```python
from build123d import *
from build123d.topology import SkipClean

# Parameters (mm, degrees)
SKETCH1_R           = 30
BOSS_EXTRUDE1_DEPTH = 20
SKETCH2_R           = 27
CUT_EXTRUDE1_DEPTH  = 7
CUT_EXTRUDE2_START  = -9
SKETCH3_R           = 27
CUT_EXTRUDE2_DEPTH  = 9
SKETCH4_R           = 6
SKETCH4_R_2         = 4
BOSS_EXTRUDE2_DEPTH = 18
BOSS_EXTRUDE3_START = 2
SKETCH5_R           = 6
BOSS_EXTRUDE3_DEPTH = 2
CUT_EXTRUDE7_START  = -42
SKETCH6_R           = 4
CUT_EXTRUDE7_DEPTH  = 42
SKETCH7_W           = 3
SKETCH7_H           = 2
BOSS_EXTRUDE4_DEPTH = 20
CIRPATTERN1_COUNT   = 25


with BuildPart() as part:
    # Sketch1 → Boss-Extrude1 (new body)
    with BuildSketch(Plane.XY):
        Circle(SKETCH1_R)
    extrude(amount=BOSS_EXTRUDE1_DEPTH)

    # Sketch2 → Cut-Extrude1 (cut)
    with BuildSketch(Plane.XY.offset(20)):
        Circle(SKETCH2_R)
    extrude(amount=-CUT_EXTRUDE1_DEPTH, mode=Mode.SUBTRACT)

    # Sketch3 → Cut-Extrude2 (cut)
    with BuildSketch(Plane(origin=(0, 0, 0), x_dir=(-1, 0, 0), z_dir=(0, 0, -1)).offset(CUT_EXTRUDE2_START)):
        with Locations(Location((0, 0, 0), (0, 0, 180))):
            Circle(SKETCH3_R)
    extrude(amount=CUT_EXTRUDE2_DEPTH, mode=Mode.SUBTRACT)

    # Sketch4 → Boss-Extrude2 (add)
    with BuildSketch(Plane.XY.offset(13)):
        Circle(SKETCH4_R)
        Circle(SKETCH4_R_2, mode=Mode.SUBTRACT)
    extrude(amount=BOSS_EXTRUDE2_DEPTH)

    # Sketch5 → Boss-Extrude3 (add)
    with BuildSketch(Plane(origin=(0, 0, 9), x_dir=(-1, 0, 0), z_dir=(0, 0, -1)).offset(BOSS_EXTRUDE3_START)):
        with Locations(Location((0, 0, 0), (0, 0, 180))):
            Circle(SKETCH5_R)
    extrude(amount=-BOSS_EXTRUDE3_DEPTH)

    # Sketch6 → Cut-Extrude7 (cut)
    with SkipClean():  # the faces are left unmerged after this step: merging them gives an invalid solid
        with BuildSketch(Plane.XY.offset(31).offset(CUT_EXTRUDE7_START)):
            with Locations(Location((0, 0, 0), (0, 0, 180))):
                Circle(SKETCH6_R)
        extrude(amount=CUT_EXTRUDE7_DEPTH, mode=Mode.SUBTRACT)
    add(part.part.scale(1), mode=Mode.REPLACE)  # the faces are merged on a copy

    # Sketch7 → Boss-Extrude4 (add)
    with BuildSketch(Plane.XY.offset(20)):
        with Locations((0, 30.891402014)):
            Rectangle(SKETCH7_W, SKETCH7_H)
    boss_extrude4 = extrude(amount=-BOSS_EXTRUDE4_DEPTH)

    # CirPattern1: Boss-Extrude4 ×25 about axis
    cirpattern1_axis = Axis((0, 0, 0), (0, 0, 1))
    for i in range(1, CIRPATTERN1_COUNT):
        add(boss_extrude4.rotate(cirpattern1_axis, i * 360 / CIRPATTERN1_COUNT))


solid = part.part
```
The model under review builds one solid part; all positions refer to its coordinate system, in mm. A direction names the side the tool comes from. Coordinates: 2 decimals unless noted, no trailing zeros. Write each loop counter-clockwise with the first axis right and the second up, starting at its lowest first coordinate (ties: lowest second). Pieces come first, ordered by that corner, then holes. Notation, with made-up numbers: (50, 7.5) - (65, 7.5) arc R14 ccw to (65, 34.5) - close; hole circle Ø8 at (74, -32.75). An arc over 180 degrees is marked (long way). Write item = value, one per line.
(1) For line 1 (Y direction, x = 0, z = 16.75); line 2 (Y direction, x = -16.5, z = 14); line 3 (Z direction, x = -16, y = 21.5), list the stretches that pass through material, from the lowest coordinate up. Write a range as [from, to].
Result sheet:
line_1 = [-30, -27], [-6, -4], [4, 6], [27, 31.89]
line_2 = [-25.26, -21.37], [21.37, 25.05], [26.9, 27.32]
line_3 = [9, 13]
(2) For P1, Ø8, axis at x = 24, y = 1.5, coming from the -Z side; P2, Ø1, axis at x = 4.5, z = 17, coming from the +Y side; P3, Ø6, axis at x = 2, y = 1.5, coming from the -Z side; P4, Ø6, axis at y = -15.5, z = 11, coming from the -X side, all flat-tipped, find the tip position at first contact; note any pin that passes through.
Result sheet:
P1 = 0
P2 = 29.73
P3 = 7
P4 = -29.36
(3) Consider section B-B, the plane z = 15. State how many separate pieces and enclosed holes the cut face has, then the cut area to 3 significant figures.
Result sheet:
separate_pieces = 2
enclosed_holes = 2
area = 743 mm^2
(4) Machinability: for faces 1 (the face through (-0.4, 6.4, 13)), 2 (the face through (-23.095, 19.147, 9.86)), 3 (the face through (-12.775, -28.19, 10.14)), 4 (the face through (30.65, -4.32, 10.14)), which of the approach directions +Z, -Z, +X, -X, +Y, -Y give a long, thin tool a straight path to every point of the face, cutting with its end or side? Answer none if there is none.
Result sheet:
face_1 = +Z
face_2 = +Z, -Z
face_3 = +Z, -Z, -X
face_4 = +Z, -Z, +X
(5) Consider section A-A, the plane x = 0. Give the boundary of the cut face in (y, z), then the cut area to 3 significant figures.
Result sheet:
outline = (-30, 0) - (-27, 0) - (-27, 9) - (-6, 9) - (-6, 7) - (-4, 7) - (-4, 31) - (-6, 31) - (-6, 13) - (-27, 13) - (-27, 20) - (-30, 20) - close; (4, 7) - (6, 7) - (6, 9) - (27, 9) - (27, 0) - (31.89, 0) - (31.89, 20) - (27, 20) - (27, 13) - (6, 13) - (6, 31) - (4, 31) - close
area = 422 mm^2
(6) Consider section D-D, the plane z = 26. Give the boundary of the cut face in (x, y).
Result sheet:
outline = circle Ø12 at (0, 0); hole circle Ø8 at (0, 0)
(7) Mouldability with a two-part tool opening along Y and no side actions: class faces 5 (the face through (-24.775, -18.549, 10.14)), 6 (the face through (-9.985, -29.295, 10.14)), 7 (the face through (15.345, 27.957, 10.14)), 8 (the face through (18, 24, 10)) as pulls with the +Y half, pulls with the -Y half, needs draft (parallel to the pull), parting line crosses it, or undercut.
Result sheet:
face_5 = undercut
face_6 = pulls with the -Y half
face_7 = pulls with the +Y half
face_8 = undercut
(8) Consider section C-C, the plane y = -22.5. Give the boundary of the cut face in (x, z), then the cut area to 3 significant figures.
Result sheet:
outline = (-19.84, 0) - (-14.92, 0) - (-14.92, 9) - (14.92, 9) - (14.92, 0) - (19.84, 0) - (19.84, 20) - (14.92, 20) - (14.92, 13) - (-14.92, 13) - (-14.92, 20) - (-19.84, 20) - close
area = 316 mm^2
